Source: CAD feature listing. Evaluate the final solid. Frame: model axes, mm. A direction names the side the tool comes from. Give positions to 0.01 mm unless a question says otherwise; leave off trailing zeros. Write each loop counter-clockwise with the first axis right and the second up, starting at its lowest first coordinate (ties: lowest second). Pieces come first, ordered by that corner, then holes. Notation, with made-up numbers: M -4,63.5 L 24,63.5 A14 cw 24,78.5 Z; hole C 44.25,64.25 d2. An arc over 180 degrees is marked long. Use CSV: the item, a comma, the result in double quotes. Start each with the question number.
from build123d import *

# Parameters (mm, degrees)
F0_R      = 20.001471
F1_DEPTH  = 17
F2_R      = 18.001471
F2_R_2    = 14.001471
F3_DEPTH  = 15
F3_FACE_R = 14.001471
F4_DEPTH  = 6
F6_DEPTH  = 25
F7_R      = 12.5
F8_DEPTH  = 10
F9_R      = 5
F10_DEPTH = 1
F11_R     = 2.5
F12_DEPTH = 8
F13_R     = 1.5
F14_DEPTH = 6


with BuildPart() as f1:
    # F0 (on Right) → F1 (new body)
    with BuildSketch(Plane.YZ):
        Circle(F0_R)
    extrude(amount=F1_DEPTH)

    # F2 (on face) → F3 (cut)
    with BuildSketch(Plane(origin=(0, 0, 0), x_dir=(0, -1, 0), z_dir=(-1, 0, 0))):
        Circle(F2_R)
        with BuildLine():
            ThreePointArc((0, -17.501471), (-1.5, -16.001471), (0, -14.501471))
            ThreePointArc((0, -14.501471), (1.06066, -14.940811), (1.5, -16.001471))
            ThreePointArc((1.5, -16.001471), (1.06066, -17.062132), (0, -17.501471))
        make_face(mode=Mode.SUBTRACT)
        with BuildLine():
            ThreePointArc((-14.501471, 0), (-16.001471, -1.5), (-17.501471, 0))
            ThreePointArc((-17.501471, 0), (-16.001471, 1.5), (-14.501471, 0))
        make_face(mode=Mode.SUBTRACT)
        Circle(F2_R_2, mode=Mode.SUBTRACT)
        with BuildLine():
            ThreePointArc((17.501471, 0), (16.001471, -1.5), (14.501471, 0))
            ThreePointArc((14.501471, 0), (16.001471, 1.5), (17.501471, 0))
        make_face(mode=Mode.SUBTRACT)
        with BuildLine():
            ThreePointArc((0, 14.501471), (-1.5, 16.001471), (0, 17.501471))
            ThreePointArc((0, 17.501471), (1.06066, 17.062132), (1.5, 16.001471))
            ThreePointArc((1.5, 16.001471), (1.06066, 14.940811), (0, 14.501471))
        make_face(mode=Mode.SUBTRACT)
    extrude(amount=-F3_DEPTH, mode=Mode.SUBTRACT)

    # F3_face (on face) → F4 (cut)
    with BuildSketch(Plane(origin=(0, 0, 0), x_dir=(0, 1, 0), z_dir=(-1, 0, 0))):
        Circle(F3_FACE_R)
    extrude(amount=-F4_DEPTH, mode=Mode.SUBTRACT)

    # F5 (on face) → F6 (cut)
    with BuildSketch(Plane(origin=(6, 0, 0), x_dir=(0, -1, 0), z_dir=(-1, 0, 0))):
        with BuildLine():
            Line((-11.06208, -4.654644), (-4.880678, -1.08581))
            ThreePointArc((-4.880678, -1.08581), (-4.993956, 0.245766), (-4.750481, 1.559784))
            Line((-4.750481, 1.559784), (-10.551599, 5.71831))
            ThreePointArc((-10.551599, 5.71831), (-11.986965, 0.58991), (-11.06208, -4.654644))
        make_face()
        with BuildLine():
            ThreePointArc((-3.002631, 3.998025), (-2.284139, 4.447776), (-1.5, 4.769696))
            Line((-1.5, 4.769696), (-1.5, 11.907364))
            ThreePointArc((-1.5, 11.907364), (-5.482605, 10.675971), (-8.803749, 8.156551))
            Line((-8.803749, 8.156551), (-3.002631, 3.998025))
        make_face()
        with BuildLine():
            ThreePointArc((1.5, 4.769696), (2.5, 4.330127), (3.380678, 3.683886))
            Line((3.380678, 3.683886), (9.56208, 7.25272))
            ThreePointArc((9.56208, 7.25272), (6.000736, 10.393579), (1.5, 11.907364))
            Line((1.5, 11.907364), (1.5, 4.769696))
        make_face()
        with BuildLine():
            ThreePointArc((4.880678, 1.08581), (4.97008, 0.546173), (5, 0))
            ThreePointArc((5, 0), (4.937226, -0.789808), (4.750481, -1.559784))
            Line((4.750481, -1.559784), (10.551599, -5.71831))
            ThreePointArc((10.551599, -5.71831), (11.633358, -2.949627), (12.001471, 0))
            ThreePointArc((12.001471, 0), (11.76428, 2.374245), (11.06208, 4.654644))
            Line((11.06208, 4.654644), (4.880678, 1.08581))
        make_face()
        with BuildLine():
            Line((8.803749, -8.156551), (3.002631, -3.998025))
            ThreePointArc((3.002631, -3.998025), (2.284139, -4.447776), (1.5, -4.769696))
            Line((1.5, -4.769696), (1.5, -11.907364))
            ThreePointArc((1.5, -11.907364), (5.482605, -10.675971), (8.803749, -8.156551))
        make_face()
        with BuildLine():
            Line((-1.5, -11.907364), (-1.5, -4.769696))
            ThreePointArc((-1.5, -4.769696), (-2.5, -4.330127), (-3.380678, -3.683886))
            Line((-3.380678, -3.683886), (-9.56208, -7.25272))
            ThreePointArc((-9.56208, -7.25272), (-6.000736, -10.393579), (-1.5, -11.907364))
        make_face()
    extrude(amount=-F6_DEPTH, mode=Mode.SUBTRACT)

    # F7 (on face) → F8 (cut)
    with BuildSketch(Plane.YZ.offset(17)):
        Circle(F7_R)
    extrude(amount=-F8_DEPTH, mode=Mode.SUBTRACT)

    # F9 (on face) → F10 (join)
    with BuildSketch(Plane(origin=(6, 0, 0), x_dir=(0, -1, 0), z_dir=(-1, 0, 0))):
        Circle(F9_R)
    extrude(amount=F10_DEPTH)

    # F11 (on face) → F12 (join)
    with BuildSketch(Plane(origin=(5, 0, 0), x_dir=(0, -1, 0), z_dir=(-1, 0, 0))):
        Circle(F11_R)
    extrude(amount=F12_DEPTH)

    # F13 (on face) → F14 (cut)
    with BuildSketch(Plane(origin=(-3, 0, 0), x_dir=(0, -1, 0), z_dir=(-1, 0, 0))):
        Circle(F13_R)
    extrude(amount=-F14_DEPTH, mode=Mode.SUBTRACT)


solid = f1.part
Item 1: Material intervals for probe 1 along Z at (x, y) = (-1.65, 0); probe 2 along Z at (x, y) = (12, -9.5); probe 3 along Y at (x, z) = (12, 15), sorted ascending.
Item 2: Contact query for flat-ended pins moving along their axis: pin 1 Ø5 at (y, z) = (-2, 4) entering from +X; pin 2 Ø1.1 at (x, z) = (6.5, -8) entering from +Y; pin 3 Ø0.9 at (y, z) = (0.5, 0.5) entering from -X. Output: stop coordinate, or through.
Item 3: Pull-direction query (Z, two-part tool) for faces 6 (the flat face through (0, 0, -16)), 7 (the cylindrical face through (6.493, 11.983, 0.665)); classes: released by +Z, released by -Z, zero draft, split by the parting line, or undercut.
Item 4: Section C-C (x = -1). Return the cut outline in (y, z), plus the area to 3 significant figures.
Item 5: Section B-B (y = 7). Return the cut outline in (x, z), plus the area to 3 significant figures.
Item 6: Section D-D (z = -0.5). State how many separate pieces and enclosed holes the cut face has, plus the area to 3 significant figures.
Item 7: Set-up query: faces 1 (the cylindrical face through (12.07, 11.923, 3.755)), 2 (the cylindrical face through (7.4, -17.17, 5.41)), 3 (the flat face through (17, -9, -9)), 4 (the flat face through (0, 0, 16)), 5 (the flat face through (6.5, 7.6, 3.6)). Return all of +Z, -Z, +X, -X, +Y, -Y with unobstructed straight access to the full face (end or side cutting, diameter ignored); none if empty.
Item 8: Section A-A (x = 12). Return the cut outline in (y, z), plus the area to 3 significant figures.
Output values:
1,probe 1,"z = -2.5 to -1.5, 1.5 to 2.5"
1,probe 2,"z = -17.6 to -15.29, -10.29 to -8.12, 8.12 to 10.29, 15.29 to 17.6"
1,probe 3,"y = -13.23 to -9.95, -1.12 to 1.12, 9.95 to 13.23"
2,pin 1,"stops at x = 7"
2,pin 2,"stops at y = 18.56"
2,pin 3,"stops at x = 3"
3,face 6,"zero draft"
3,face 7,"undercut"
4,outline,"C 0,0 d5; hole C 0,0 d3"
4,area,"12.6 mm2"
5,outline,"M 0,-18.74 L 17,-18.74 L 17,-10.36 L 7,-10.36 L 7,-9.75 L 6,-9.75 L 6,-12.13 L 15,-12.13 L 15,-16.58 L 0,-16.58 Z; M 0,16.58 L 15,16.58 L 15,12.13 L 6,12.13 L 6,9.75 L 7,9.75 L 7,10.36 L 17,10.36 L 17,18.74 L 0,18.74 Z; M 6,-5.77 L 7,-5.77 L 7,-2.31 L 6,-2.31 Z; M 6,3.17 L 7,3.17 L 7,6.86 L 6,6.86 Z"
5,area,"138 mm2"
6,separate pieces,"3"
6,enclosed holes,"0"
6,area,"245 mm2"
7,face 1,"+X"
7,face 2,"-X"
7,face 3,"+Z, -Z, +X, +Y, -Y"
7,face 4,"+Z, -X, +Y, -Y"
7,face 5,"+X, -X"
8,outline,"C 0,0 d40; C -16,0 d3; C 0,0 d28; M -1.5,-16 A1.5 ccw 0,-17.5 A1.5 ccw long Z; M -1.5,16 A1.5 ccw long 0,17.5 A1.5 ccw Z; C 16,0 d3; hole C 0,0 d36; hole C 0,0 d25"
8,area,"392 mm2"
